Autodesk Inventor part; units mm, degrees
ref_plane "YZ Plane" through (0, 0, 0) normal (1, 0, 0) x (0, 1, 0)
ref_plane "XZ Plane" through (0, 0, 0) normal (0, 1, 0) x (-1, 0, 0)
ref_plane "XY Plane" through (0, 0, 0) normal (0, 0, 1) x (1, 0, 0)
sketch "Sketch1" plane through (0, 0, 0) normal (0, 0, 1) x (1, 0, 0)
  line L0 (-198.2999, 0) -> (115.1427, 0)
  line L1 (0, -203.8942) -> (0, 193.807)
  circle A0 centre (0, 0) radius 53.975 construction
  circle A1 centre (0, 0) radius 19.05
  arc A2 (50.8401, -18.1268) -> (-4.087, 53.82) centre (0, 0) ccw
  line L2 (51.6197, -23.9016) -> (59.4633, -35.1034)
  arc A3 (50.8401, -18.1268) -> (51.6197, -23.9016) centre (56.8213, -20.2594) ccw
  line L3 (0, 0) -> (-57.7807, -26.9436) construction
  circle A4 centre (0, 0) radius 53.975 construction
  circle A5 centre (-95.7467, 0) radius 11.1125
  circle A6 centre (-73.1257, -37.5239) radius 14.2875
  circle A7 centre (-82.0671, 38.2685) radius 14.2875
  arc A8 (-56.7688, 67.6544) -> (-118.11, 48.895) centre (-79.7827, 33.238) ccw
  arc A9 (-118.11, -50.8) -> (-59.2151, -78.8871) centre (-77.6901, -41.8358) ccw
  arc A10 (-12.3378, -71.9752) -> (-59.2151, -78.8871) centre (-25.2121, -147.0797) ccw
  circle A11 centre (0, 0) radius 16.51 construction
  line L4 (0, 0) -> (-82.0671, 38.2685) construction
  circle A12 centre (-125.73, 34.29) radius 6.35 construction
  circle A13 centre (-125.73, -34.29) radius 6.35 construction
  line L5 (0, 0) -> (-34.422, 64.7383) construction
  line L6 (0, 0) -> (-56.7688, 67.6544) construction
  arc A14 (-127.2193, 41.2768) -> (-132.0785, 31.0144) centre (-125.73, 34.29) ccw
  arc A15 (-130.3268, 13.3001) -> (-130.3268, -13.3001) centre (-83.9357, 0) ccw
  arc A16 (-130.3268, 13.3001) -> (-132.0785, 31.0144) centre (-153.5223, 19.9501) ccw
  arc A17 (-132.0785, -31.0144) -> (-127.4503, -41.2235) centre (-125.73, -34.29) ccw
  arc A18 (-132.0785, -31.0144) -> (-130.3268, -13.3001) centre (-153.5223, -19.9501) ccw
  arc A19 (-118.11, -50.8) -> (-127.4503, -41.2235) centre (-130.5087, -53.5498) ccw
  arc A20 (-127.2193, 41.2768) -> (-118.11, 48.895) centre (-129.8669, 53.6978) ccw
  line L7 (-198.2999, 0) -> (115.1427, 0)
  line L8 (0, 193.807) -> (0, -203.8942)
  line L9 (-118.11, -50.8) -> (0, -50.8) construction
  arc A21 (-12.3378, -71.9752) -> (59.4295, -42.4357) centre (0, 0) ccw
  arc A22 (59.4295, -42.4357) -> (59.4633, -35.1034) centre (54.2617, -38.7456) ccw
  line L10 (0, 0) -> (41.8854, -59.8186) construction
  line L11 (-118.11, 48.895) -> (0, 48.895) construction
  arc A23 (-56.7688, 67.6544) -> (-4.087, 53.82) centre (-10.4031, 136.9926) ccw
  point P0 (61.9528, -38.6588)
  point P1 (-67.9722, -26.6913)
  dimension "d67" = 107.95
  dimension "d68" = 38.1
  dimension "d84" = 65
  dimension "d88" = 107.95
  dimension "d89" = 22.225
  dimension "d90" = 28.575
  dimension "d99" = 33.02
  dimension "d100" = 43.815
  dimension "d103" = 28.575
  dimension "d105" = 90.551
  dimension "d106" = 12.7
  dimension "d107" = 12.7
  dimension "d114" = 14.2875
  dimension "d115" = 14.2875
  dimension "d117" = 24.13
  dimension "d118" = 24.13
  dimension "d119" = 48.26
  dimension "d120" = 12.7
  dimension "d124" = 76.2
  dimension "d127" = 28
  dimension "d128" = 40
  dimension "d129" = 65
  dimension "d130" = 40.64
  dimension "d131" = 34.29
  dimension "d132" = 34.29
  dimension "d133" = 125.73
  dimension "d134" = 125.73
  dimension "d138" = 11.811
  dimension "d140" = 50.8
  dimension "d141" = 118.11
  dimension "d153" = 35
  dimension "d154" = 6.35
  dimension "d155" = 6.35
  dimension "d167" = 73.025
  dimension "d168" = 28.575
  dimension "d169" = 12.7
  dimension "d170" = 41.402
  dimension "d173" = 118.11
  dimension "d174" = 48.895
extrude "Base" add sketch "Sketch1" along normal mid plane 6.35 contours A15 A16 A14 A20 A8 A23 A2 L1 A1 L0 A5 | L0 A5 A1 L1 A21 A10 A9 A19 A17 A18 A15 | L1 A2 L0 A1 | A1 L0 A2 A3 L2 A22 A21 L1
sketch "Sketch2" plane through (0, 0, -3.175) normal (0, 0, -1) x (-1, 0, 0)
  arc A0 (127.4503, -41.2235) -> (132.0785, -31.0144) centre (125.73, -34.29) ccw
  arc A1 (132.0785, 31.0144) -> (127.2193, 41.2768) centre (125.73, 34.29) ccw
hole "Standoff holes to back plate" at (-125.73, 34.29, -3.175) at (-125.73, -34.29, -3.175) direction (0, 0, 1) diameter 5.1054 end through all counterbore diameter 9.779 counterbore depth 1.5875
sketch "Sketch3" plane through (0, 0, 3.175) normal (0, 0, 1) x (1, 0, 0)
  arc A0 (-12.3378, -71.9752) -> (59.4295, -42.4357) centre (0, 0) ccw
  line L0 (51.6197, -23.9016) -> (59.4633, -35.1034)
  arc A1 (50.8401, -18.1268) -> (-4.087, 53.82) centre (0, 0) ccw
  line L1 (-173.5215, 0) -> (111.013, 0)
  line L2 (0, -114.8134) -> (0, 106.2156)
  arc A2 (0, -61.5061) -> (47.1164, -39.5354) centre (0, 0) ccw
  arc A3 (52.2921, -43.8783) -> (47.1164, -39.5354) centre (49.7043, -41.7068) ccw
  arc A4 (0, -61.5061) -> (0, -68.2625) centre (0, -64.8843) ccw
  arc A5 (0, -68.2625) -> (52.2921, -43.8783) centre (0, 0) ccw
  line L3 (49.7043, -41.7068) -> (0, 0) construction
  line L4 (0, -64.8843) -> (0, 0) construction
  point P0 (-10.4819, 52.9474)
  dimension "d159" = 4.7625
  dimension "d160" = 6.7564
  dimension "d161" = 15
  dimension "d162" = 50
extrude "Tensioning Slot" cut sketch "Sketch3" against normal through all contours A2 A3 A5 L2 | L2 A4
sketch "Sketch4" plane through (0, 0, 3.175) normal (0, 0, 1) x (1, 0, 0)
  arc A0 (50.8401, -18.1268) -> (-4.087, 53.82) centre (0, 0) ccw
  arc A1 (-12.3378, -71.9752) -> (59.4295, -42.4357) centre (0, 0) ccw
  line L0 (-173.5215, 0) -> (111.013, 0)
  line L1 (0, -114.8134) -> (0, 106.2156)
  arc A2 (41.8111, 7.3724) -> (48.4649, 8.5457) centre (45.138, 7.959) ccw
  arc A3 (4.2892, 49.0252) -> (3.7003, 42.2945) centre (3.9947, 45.6599) ccw
  arc A4 (41.8111, 7.3724) -> (3.7003, 42.2945) centre (0, 0) ccw
  arc A5 (48.4649, 8.5457) -> (4.2892, 49.0252) centre (0, 0) ccw
  line L2 (0, 0) -> (3.9947, 45.6599) construction
  line L3 (0, 0) -> (45.138, 7.959) construction
  dimension "d181" = 4.7625
  dimension "d182" = 6.7564
  dimension "d183" = 75
  dimension "d187" = 10
extrude "Tensioning Slot:2" cut sketch "Sketch4" against normal through all contours A4 A3 A5 A2
equation "\"d132\" = d131"
equation "\"d134\" = d133"
properties part number "front plate"
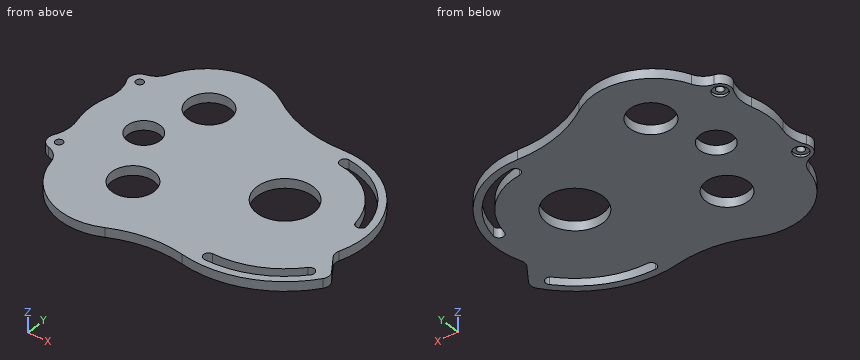
Could you check a few things on this model? Use its own coordinates, in mm. Coordinates: 2 decimals unless noted, no trailing zeros. Order: outer loops, then holes, each group sorted by start corner. A loop starts at its lowest first (then second) coordinate and runs counter-clockwise, first axis right, second up. Notation, with made-up numbers: M -13.75,82.5 L -4.75,82.5 A11 ccw -4.75,89.5 Z; hole C 67.25,74 d5. An arc over 180 degrees is marked long. Use one line per item in the form item = value. Start each with the question number.
1. Please list where these lines run through material, in increasing order: line 1 (X direction, y = 0, z = -1); line 2 (Y direction, x = -125.73, z = -2.45); line 3 (X direction, y = 14, z = -1.25).
2. Suppose I cut it at D-D on z = 1. Count the separate pieces of the cut face and the enclosed holes in it, then the cut area to 3 significant figures.
3. Suppose I cut it at A-A on y = 0. Write out the boundary of the cut face in (x, z) (3 decimals), then the cut area to 3 significant figures.
4. Suppose I cut it at C-C on y = -64. Write out the boundary of the cut face in (x, z) (3 decimals).
5. For pin 1 (1.5 mm diameter, centred on y = -14.5, z = 2, fed in from +X), with a flat end and sliding along its axis, tell me the tip position at first contact or that it passes through.
6. Suppose I cut it at B-B on x = 10.5. Write out the boundary of the cut face in (y, z) (3 decimals), then the cut area to 3 significant figures.
Geometry says:
q1.line_1 = -132.2 to -106.86, -84.63 to -19.05, 19.05 to 53.97
q1.line_2 = -41.78 to -39.18, -29.4 to 29.4, 39.18 to 41.69
q1.line_3 = -130.14 to -12.92, 12.92 to 40.08, 47.18 to 52.13
q2.separate_pieces = 1
q2.enclosed_holes = 8
q2.area = 19,600 mm^2
q3.outline = M -132.196,-3.175 L -106.859,-3.175 L -106.859,3.175 L -132.196,3.175 Z; M -84.634,-3.175 L -19.05,-3.175 L -19.05,3.175 L -84.634,3.175 Z; M 19.05,-3.175 L 53.975,-3.175 L 53.975,3.175 L 19.05,3.175 Z
q3.area = 799 mm^2
q4.outline = M -112.66,-3.175 L -3.26,-3.175 L -3.26,3.175 L -112.66,3.175 Z; M 23.744,-3.175 L 35.166,-3.175 L 35.166,3.175 L 23.744,3.175 Z
q5.pin_1 = 52.19
q6.outline = M -72.266,-3.175 L -67.45,-3.175 L -67.45,3.175 L -72.266,3.175 Z; M -60.603,-3.175 L -15.895,-3.175 L -15.895,3.175 L -60.603,3.175 Z; M 15.895,-3.175 L 41.137,-3.175 L 41.137,3.175 L 15.895,3.175 Z; M 48.079,-3.175 L 52.944,-3.175 L 52.944,3.175 L 48.079,3.175 Z
q6.area = 506 mm^2
